Read the model definition and answer for the solid it produces. Units are mm, in the model's axes. A direction names the side the tool comes from. Coordinates: 2 decimals unless noted, no trailing zeros. Loops run counter-clockwise (first coordinate to the right, second up) from the corner with the lowest first, then second, coordinate; pieces in that order, holes last. Notation, with made-up numbers: M -8,16.25 L 30,16.25 A15 cw 30,27.25 Z; hole C 78.5,-33.5 d1. An arc over 180 degrees is marked long. Put each result on its own line as item: value.
from build123d import *

# Parameters (mm, degrees)
F0_R     = 7.5
F1_DEPTH = 25
F2_R     = 2.75
F3_DEPTH = 10
F4_W     = 4
F4_H     = 15
F5_DEPTH = 10


with BuildPart() as f1:
    # F0 (on Front) → F1 (new body)
    with BuildSketch(Plane.XZ):
        Circle(F0_R)
    extrude(amount=F1_DEPTH)

    # F2 (on face) → F3 (cut)
    with BuildSketch(Plane.XZ.offset(25)):
        Circle(F2_R)
    extrude(amount=-F3_DEPTH, mode=Mode.SUBTRACT)

    # F4 (on face) → F5 (cut)
    with BuildSketch(Plane(origin=(0, 0, 0), x_dir=(-1, 0, 0), z_dir=(0, 1, 0))):
        Rectangle(F4_W, F4_H)
    extrude(amount=-F5_DEPTH, mode=Mode.SUBTRACT)


solid = f1.part
1) Given pin 1 Ø4.5 at (x, z) = (0, 0) entering from +Y; pin 2 Ø3 at (x, z) = (0, 0.5) entering from +Y; pin 3 Ø3 at (y, z) = (-7.5, 2) entering from -X; pin 4 Ø1.5 at (y, z) = (-14.5, 1.5) entering from +X, each flat-ended and moving along its own axis, determine where each tip first touches the part or whether it passes through.
Answer list:
pin 1: stops at y = 0
pin 2: stops at y = -10
pin 3: stops at x = -7.48
pin 4: stops at x = 7.46
2) Straight lines are drawn through the part: line 1 (Z direction, x = 0, y = -23); line 2 (Y direction, x = -0.5, z = -4.25); line 3 (X direction, y = -23.25, z = -1). For each, find the intervals that lie inside material, in ascending order. Write a range as [from, to].
Answer list:
line 1: z = [-7.5, -2.75], [2.75, 7.5]
line 2: y = [-25, -10]
line 3: x = [-7.43, -2.56], [2.56, 7.43]
3) Find section C-C, the plane y = -1.5. Write down the section's boundary in (x, z).
Answer list:
outline: M -2,-7.23 L -2,7.23 A7.5 ccw Z; M 2,-7.23 A7.5 ccw 2,7.23 Z
4) Find section A-A, the plane x = 0. Write down the section's boundary in (y, z), plus the area to 3 significant figures.
Answer list:
outline: M -25,-7.5 L -10,-7.5 L -10,7.5 L -25,7.5 L -25,2.75 L -15,2.75 L -15,-2.75 L -25,-2.75 Z
area: 170 mm^2
5) Which of the six approach directions +Z, -Z, +X, -X, +Y, -Y give full straight-line access (tool end or side, diameter ignored) to faces 1 (the flat face through (0, -15, 0)), 2 (the flat face through (-2, -5, 0)), 3 (the flat face through (4, 0, 0))?
Answer list:
face 1: -Y
face 2: +Z, -Z, +Y
face 3: +Z, -Z, +X, -X, +Y
6) Determine the mould class of faces 4 (the flat face through (-4, 0, 0)), 5 (the cylindrical face through (-0.596, -20.07, -2.685)), 6 (the cylindrical face through (7.154, -12.325, 2.253)) for opening direction X: released by +X, released by -X, zero draft, split by the parting line, or undercut.
Answer list:
face 4: zero draft
face 5: undercut
face 6: split by the parting line
7) Find section B-B, the plane z = 0. Write down the section's boundary in (x, y), plus the area to 3 significant figures.
Answer list:
outline: M -7.5,-25 L -2.75,-25 L -2.75,-15 L 2.75,-15 L 2.75,-25 L 7.5,-25 L 7.5,0 L 2,0 L 2,-10 L -2,-10 L -2,0 L -7.5,0 Z
area: 280 mm^2
8) Find section D-D, the plane z = -4.5. Write down the section's boundary in (x, y), plus the area to 3 significant figures.
Answer list:
outline: M -6,-25 L 6,-25 L 6,0 L 2,0 L 2,-10 L -2,-10 L -2,0 L -6,0 Z
area: 260 mm^2
